The listing builds one solid part. Answer for the finished solid, in the listing's coordinates (mm). A direction names the side the tool comes from. Give positions to 0.01 mm unless a question says otherwise; leave off trailing zeros. Order: outer loops, then holes, each group sorted by start corner. A loop starts at its lowest first (then second) coordinate and runs counter-clockwise, first axis right, second up.
```python
from build123d import *

# Parameters (mm, degrees)
SKETCH_1_R      = 1.6
EXTRUDE_1_DEPTH = 2
SKETCH_3_R      = 1.6
EXTRUDE_2_DEPTH = 1.5
FILLET_2_R      = 3


with BuildPart() as part:
    # ｽｹｯﾁ1 → ﾎﾞｽ - 押し出し1 (new body)
    with BuildSketch(Plane.XY):
        Polygon((-27.32233047, -13.180194847), (-20.251262658, -20.251262658), (0, 0), (20.628932188, 0), (20.628932188, 10), (-4.142135624, 10), align=None)
        with Locations((3.128932188, 5)):
            Circle(SKETCH_1_R, mode=Mode.SUBTRACT)
        with Locations((15.628932188, 5)):
            Circle(SKETCH_1_R, mode=Mode.SUBTRACT)
        with Locations((-20.251262658, -13.180194847)):
            Circle(SKETCH_1_R, mode=Mode.SUBTRACT)
        with Locations((-9.644660941, -2.573593129)):
            Circle(SKETCH_1_R, mode=Mode.SUBTRACT)
    extrude(amount=EXTRUDE_1_DEPTH)

    # ｽｹｯﾁ3 → ﾎﾞｽ - 押し出し2 (add)
    with BuildSketch(Plane.XY.offset(2)):
        Polygon((13.028932188, 0), (5.656349186, -7.372583002), (12.727416998, -14.443650814), (27.171067812, 0), (27.171067812, 10), (20.628932188, 10), (20.628932188, 0), align=None)
        with Locations((12.727416998, -7.372583002)):
            Circle(SKETCH_3_R, mode=Mode.SUBTRACT)
    extrude(amount=-EXTRUDE_2_DEPTH)

    # ﾌｨﾚｯﾄ2
    fillet_2_edges = [part.edges().sort_by_distance(p)[0] for p in [
        (-4.142135624, 10, 1),
        (0, 0, 1),
        (-20.251262658, -20.251262658, 1),
        (-27.32233047, -13.180194847, 1),
        (27.171067812, 10, 1.25),
        (27.171067812, 0, 1.25),
        (12.727416998, -14.443650814, 1.25),
        (5.656349186, -7.372583002, 1.25),
        (13.028932188, 0, 1.25),
    ]]
    fillet(fillet_2_edges, radius=FILLET_2_R)


solid = part.part
```
1) A tool of negligible diameter and unlimited length cuts with its end or side. For faces 4 (the flat face through (6.5, 0, 0.3)), 5 (the cylindrical face through (6.9, -7.3, 1.2)), 6 (the flat face through (9.172, -10.888, 1.26)), from which of +Z, -Z, +X, -X, +Y, -Y can it reach the whole face along a straight path? Write none if from no direction.
Geometry says:
face 4: -Z, -Y
face 5: +Z, -Z
face 6: +Z, -Z, -Y
2) Find section B-B (y = 6). Write down the section's boundary in (x, z).
Geometry says:
outline: (-8.14, 0) - (1.88, 0) - (1.88, 2) - (-8.14, 2) - close; (4.38, 0) - (14.38, 0) - (14.38, 2) - (4.38, 2) - close; (16.88, 0) - (20.63, 0) - (20.63, 0.5) - (27.17, 0.5) - (27.17, 2) - (16.88, 2) - close
3) Given P1, Ø1, axis at x = 8, z = 1.5, coming from the -Y side; P2, Ø2.5, axis at x = -20.25, y = -13.18, coming from the +Z side; P3, Ø0.6, axis at y = 2.5, z = 0, coming from the +X side, each flat-ended and moving along its own axis, determine where each tip first touches the part or whether it passes through.
Geometry says:
P1: stops at y = -10.22
P2: passes through
P3: stops at x = 20.63
4) Find section C-C (z = 1.25). Write down the section's boundary in (x, y), then the cut area to 3 significant figures.
Geometry says:
outline: (-25.2, -15.3) - (-22.37, -18.13) arc R3 ccw to (-18.13, -18.13) - (-0.88, -0.88) arc R3 cw to (1.24, 0) - (5.79, 0) arc R3 cw to (7.91, -5.12) - (7.78, -5.25) arc R3 ccw to (7.78, -9.49) - (10.61, -12.32) arc R3 ccw to (14.85, -12.32) - (26.29, -0.88) arc R3 ccw to (27.17, 1.24) - (27.17, 7) arc R3 ccw to (24.17, 10) - (-2.9, 10) arc R3 ccw to (-5.02, 9.12) - (-25.2, -11.06) arc R3 ccw to start; hole circle Ø3.2 at (-20.25, -13.18); hole circle Ø3.2 at (-9.64, -2.57); hole circle Ø3.2 at (3.13, 5); hole circle Ø3.2 at (12.73, -7.37); hole circle Ø3.2 at (15.63, 5)
area: 715 mm2
5) Find section D-D (x = 0). Write down the section's boundary in (y, z), then the cut area to 3 significant figures.
Geometry says:
outline: (-0.27, 0) - (10, 0) - (10, 2) - (-0.27, 2) - close
area: 20.5 mm2
6) For a pull along X with two mould halves and no side action, classify faces 1 (the cylindrical face through (26.95, 0.11, 1.24)), 2 (the cylindrical face through (11.46, -8.35, 1.26)), 3 (the cylindrical face through (-20, -19, 1)) as +X half, -X half, draft (parallel to the pull), parting line (faces both ways), or undercut.
Geometry says:
face 1: +X half
face 2: undercut
face 3: parting line
7) Straight lines are drawn through the part: probe 1 along X at (y, z) = (-8, 0.85); probe 2 along Y at (x, z) = (18.5, 0.3); probe 3 along Z at (x, y) = (23, 1). For each, find the intervals that lie inside material, in ascending order.
Geometry says:
probe 1: x = -22.14 to -8, 6.97 to 11.26, 14.2 to 19.17
probe 2: y = 0 to 10
probe 3: z = 0.5 to 2
8) Find section A-A (x = -21). Write down the section's boundary in (y, z), then the cut area to 3 significant figures.
Geometry says:
outline: (-18.91, 0) - (-14.59, 0) - (-14.59, 2) - (-18.91, 2) - close; (-11.77, 0) - (-6.86, 0) - (-6.86, 2) - (-11.77, 2) - close
area: 18.5 mm2
